```python
from build123d import *

# Parameters (mm, degrees)
PAD_DEPTH       = 45
SKETCH001_R     = 1.6
POCKET_DEPTH    = 5.68
SKETCH002_R     = 2.4
SKETCH002_R_2   = 1.6
PAD001_DEPTH    = 4
SKETCH003_R     = 1.6
POCKET001_DEPTH = 2.4
PAD002_DEPTH    = 2.4
SKETCH004_R     = 3.05
POCKET002_DEPTH = 9.68
SKETCH005_R     = 3.05
PAD003_DEPTH    = 1
SKETCH006_R     = 1.6
POCKET003_DEPTH = 5.681
POCKET004_DEPTH = 2.3
SKETCH008_R     = 2.75
POCKET005_DEPTH = 1.5
CHAMFER_SIZE    = 1


with BuildPart() as part:
    # Sketch → Pad (new body)
    with BuildSketch(Plane.XY):
        Polygon((2.94, -2.84), (-2.94, -2.84), (-5.44, -0.52), (-5.44, 1.16), (-2.94, 1.16), (-2.94, 2.84), (2.94, 2.84), (2.94, 1.16), (5.44, 1.16), (5.44, -0.52), align=None)
    extrude(amount=PAD_DEPTH)

    # Sketch001 (on Face6 of Pad) → Pocket (cut)
    with BuildSketch(Plane(origin=(0, 2.84, 0), x_dir=(-1, 0, 0), z_dir=(0, 1, 0))):
        with Locations((0, 22.5)):
            Circle(SKETCH001_R)
    extrude(amount=-POCKET_DEPTH, mode=Mode.SUBTRACT)

    # Sketch002 (on Face11 of Pocket) → Pad001 (join)
    with BuildSketch(Plane(origin=(0, 2.84, 0), x_dir=(-1, 0, 0), z_dir=(0, 1, 0))):
        with Locations((0, 22.5)):
            Circle(SKETCH002_R)
        with Locations((0, 22.5)):
            Circle(SKETCH002_R_2, mode=Mode.SUBTRACT)
    extrude(amount=PAD001_DEPTH)

    # Sketch003 (on Face1 of Pad001) → Pocket001 (cut)
    with BuildSketch(Plane.XZ.offset(2.84)):
        Polygon((0, 19.186009), (2.87, 20.843005), (2.87, 24.156995), (0, 25.813991), (-2.87, 24.156995), (-2.87, 20.843005), align=None)
        with Locations((0, 22.5)):
            Circle(SKETCH003_R, mode=Mode.SUBTRACT)
    extrude(amount=-POCKET001_DEPTH, mode=Mode.SUBTRACT)

    # Pocket001 Face19 → Pad002 (add)
    with BuildSketch(Plane(origin=(0, -0.44, 22.5), x_dir=(-1, 0, 0), z_dir=(0, -1, 0))):
        Polygon((0, 3.313991), (-2.87, 1.656995), (-2.87, -1.656995), (0, -3.313991), (2.87, -1.656995), (2.87, 1.656995), align=None)
        with BuildLine():
            ThreePointArc((1.6, 0), (0, -1.6), (-1.6, 0))
            ThreePointArc((-1.6, 0), (0, 1.6), (1.6, 0))
        make_face(mode=Mode.SUBTRACT)
    extrude(amount=PAD002_DEPTH)

    # Sketch004 (on Face16 of Pad001) → Pocket002 (cut)
    with BuildSketch(Plane(origin=(0, 6.84, 0), x_dir=(-1, 0, 0), z_dir=(0, 1, 0))):
        with Locations((0, 22.5)):
            Circle(SKETCH004_R)
    extrude(amount=-POCKET002_DEPTH, mode=Mode.SUBTRACT)

    # Sketch005 (on Face12 of Pocket002) → Pad003 (join)
    with BuildSketch(Plane(origin=(0, 2.84, 0), x_dir=(-1, 0, 0), z_dir=(0, 1, 0))):
        with Locations((0, 22.5)):
            Circle(SKETCH005_R)
    extrude(amount=-PAD003_DEPTH)

    # Sketch006 (on Face17 of Pad003) → Pocket003 (cut, through all)
    with BuildSketch(Plane.XZ.offset(2.84)):
        with Locations((0, 39.686)):
            Circle(SKETCH006_R)
        with Locations((0, 5.314)):
            Circle(SKETCH006_R)
    extrude(amount=-POCKET003_DEPTH, mode=Mode.SUBTRACT)

    # Sketch007 (on Face1 of Pocket003) → Pocket004 (cut)
    with BuildSketch(Plane.XZ.offset(2.84)):
        Polygon((0, 36.452838), (2.8, 38.069419), (2.8, 41.302581), (0, 42.919162), (-2.8, 41.302581), (-2.8, 38.069419), align=None)
        Polygon((0, 2.080838), (2.8, 3.697419), (2.8, 6.930581), (0, 8.547162), (-2.8, 6.930581), (-2.8, 3.697419), align=None)
    extrude(amount=-POCKET004_DEPTH, mode=Mode.SUBTRACT)

    # Sketch008 (on Face41 of Pocket004) → Pocket005 (cut)
    with BuildSketch(Plane(origin=(0, 2.84, 0), x_dir=(-1, 0, 0), z_dir=(0, 1, 0))):
        with Locations((0, 39.686)):
            Circle(SKETCH008_R)
        with Locations((0, 5.314)):
            Circle(SKETCH008_R)
    extrude(amount=-POCKET005_DEPTH, mode=Mode.SUBTRACT)

    # Chamfer
    chamfer_edges = [part.edges().sort_by_distance(p)[0] for p in [
        (2.75, 1.34, 5.314),
        (2.75, 1.34, 39.686),
    ]]
    chamfer(chamfer_edges, length=CHAMFER_SIZE)


solid = part.part
```
Could you check a few things on this model? Use its own coordinates, in mm. A direction names the side the tool comes from. Coordinates: 2 decimals unless noted, no trailing zeros. Loops run counter-clockwise (first coordinate to the right, second up) from the corner with the lowest first, then second, coordinate; pieces in that order, holes last.
1) Will these pins go through, and if not, where does the flat tip stop? pin 1 Ø0.5 at (y, z) = (2, 30.5) entering from +X; pin 2 Ø3 at (x, z) = (0, 39) entering from -Y; pin 3 Ø0.8 at (y, z) = (2.5, 13) entering from -X.
Reported:
pin 1: stops at x = 2.94
pin 2: stops at y = -0.54
pin 3: stops at x = -2.94
2) Imagine slicing it at D-D (x = -4.5). List the corners of the cut face in (y, z) for me, and give its area (3 significant figures).
Reported:
outline: (-1.39, 0) - (1.16, 0) - (1.16, 45) - (-1.39, 45) - close
area: 115 mm2
3) Please list where these lines run through material, in increasing order: line 1 along Z through (x, y) = (0, 0.4); line 2 along Z through (x, y) = (0, 2.5); line 3 along Z through (x, y) = (2, -1.35).
Reported:
line 1: z = 0 to 3.71, 6.91 to 19.45, 25.55 to 38.09, 41.29 to 45
line 2: z = 0 to 2.56, 8.06 to 36.94, 42.44 to 45
line 3: z = 0 to 3.24, 7.39 to 20.2, 24.8 to 37.61, 41.76 to 45
4) Which directions (+Z, -Z, +X, -X, +Y, -Y) give clear straight access to the entire face, cutting with the end or side of a thin tool? Please do faces 1 (the face through (-3.05, 2.35, 22.49)), 2 (the face through (-4, 1.16, 22)), 3 (the face through (-1.38, -1.71, 7.75)), 4 (the face through (4.21, -1.66, 22.18)), 5 (the face through (3.05, 2.35, 22.51)).
Reported:
face 1: -X, +Y
face 2: +Z, -Z, -X, +Y
face 3: -Y
face 4: +Z, -Z, +X, -Y
face 5: +X, +Y
5) Imagine slicing it at A-A (y = 0.75). List the corners of the cut face in (x, z) for me.
Reported:
outline: (-5.44, 0) - (5.44, 0) - (5.44, 45) - (-5.44, 45) - close; hole circle Ø6.1 at (0, 22.5); hole circle Ø3.2 at (0, 5.31); hole circle Ø3.2 at (0, 39.69)
6) Imagine slicing it at C-C (z = 17.5). List the corners of the cut face in (x, y) for me, and give its area (3 significant figures).
Reported:
outline: (-5.44, -0.52) - (-2.94, -2.84) - (2.94, -2.84) - (5.44, -0.52) - (5.44, 1.16) - (2.94, 1.16) - (2.94, 2.84) - (-2.94, 2.84) - (-2.94, 1.16) - (-5.44, 1.16) - close
area: 47.6 mm2
7) Thinking about a two-plate mould opening in X: for faces 6 (the face through (-5.44, 0, 22)), 7 (the face through (-0.2, 0.4, 6.9)), 8 (the face through (0, 0, 45)), which applies, released by +X, released by -X, zero draft, split by the parting line, or undercut?
Reported:
face 6: released by -X
face 7: undercut
face 8: zero draft
8) Imagine slicing it at B-B (z = 22.5). List the corners of the cut face in (x, y) for me, and give its area (3 significant figures).
Reported:
outline: (-5.44, -0.52) - (-3.05, -2.74) - (-3.05, 1.16) - (-5.44, 1.16) - close; (-3.05, 1.84) - (3.05, 1.84) - (3.05, 2.84) - (-3.05, 2.84) - close; (3.05, -2.74) - (5.44, -0.52) - (5.44, 1.16) - (3.05, 1.16) - close
area: 19.4 mm2
